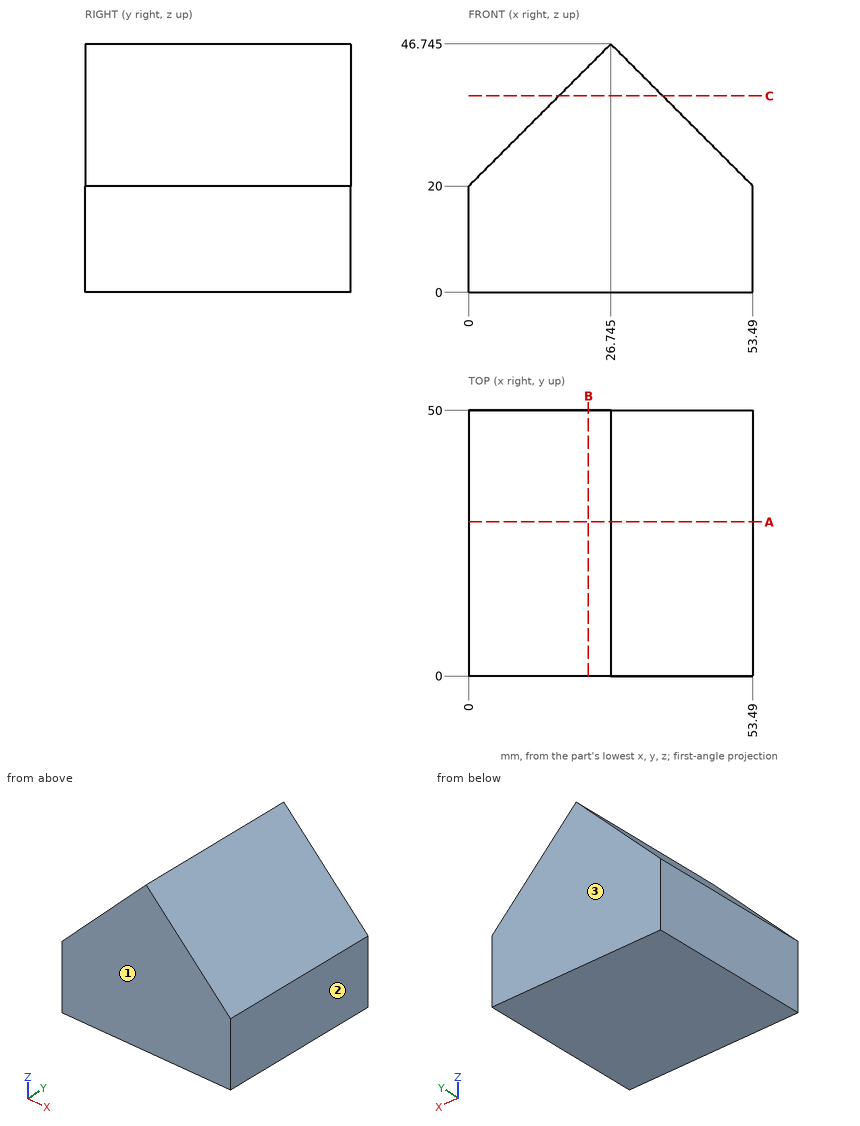
The drawing under review shows one solid part. Ordinate dimensions are in mm from its lowest x, y, z. Coordinates: 2 decimals unless noted, no trailing zeros. Order: outer loops, then holes, each group sorted by start corner. A loop starts at its lowest first (then second) coordinate and runs counter-clockwise, first axis right, second up. Notation, with made-up numbers: (28.5, 88) -> (75.5, 88) arc R21 cw to (75.5, 117) -> close; hole circle Ø1 at (-0.5, 1.25). An arc over 180 degrees is marked (long way). Return JSON: item names as keys, results as strings.
1. The part is to be moulded in two halves that separate along Y. For the marked faces 1, 2 and 3, say which applies: +Y half, -Y half, draft (parallel to the pull), parting line (faces both ways), or undercut.
Answer block:
{"face 1": "-Y half", "face 2": "draft", "face 3": "+Y half"}
2. For pin 1 Ø3 at (x, y) = (13, 30) entering from +Z, flat-tipped, find the tip position at first contact; note if it passes through.
Answer block:
{"pin 1": "z = 34.5"}
3. We need section B-B on x = 22.5. Write out the cut boundary in (y, z), and give its area (4 significant figures).
Answer block:
{"outline": "(0, 0) -> (50, 0) -> (50, 42.5) -> (0, 42.5) -> close", "area": "2,125 mm²"}
4. We need section A-A on y = 29. Write out the cut boundary in (x, z) (1 decimal).
Answer block:
{"outline": "(0, 0) -> (53.5, 0) -> (53.5, 20) -> (26.7, 46.7) -> (0, 20) -> close"}
5. For line 1 (X direction, y = 23.5, z = 21); line 2 (Z direction, x = 23.5, y = 39); line 3 (Z direction, x = 48.5, y = 27.5), list the stretches that pass through material, from the lowest coordinate up. Write a range as from..to.
Answer block:
{"line 1": "1..52.49", "line 2": "0..43.5", "line 3": "0..24.99"}
6. We need section C-C on z = 37. Write out the cut boundary in (x, y).
Answer block:
{"outline": "(17, 0) -> (36.49, 0) -> (36.49, 50) -> (17, 50) -> close"}
